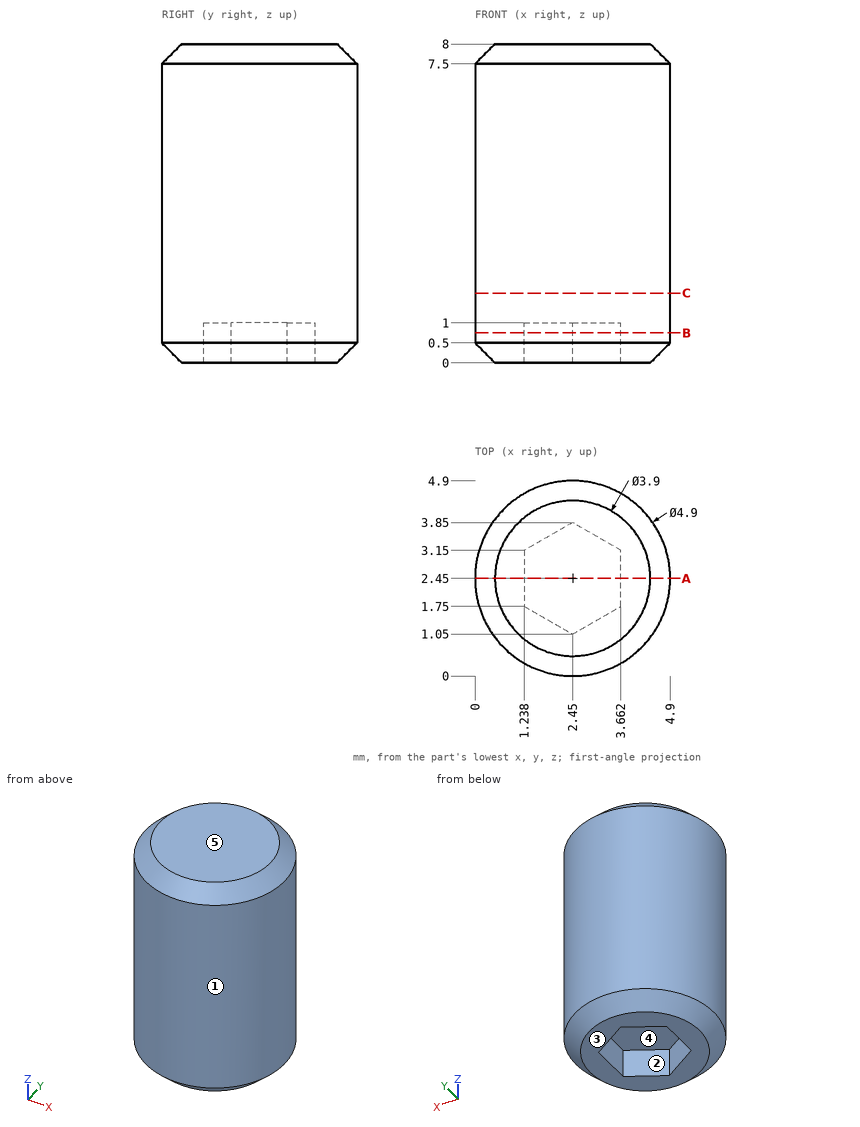
Job drawing, mm, ordinate dimensions from the low corner. One solid piece. A direction names the side the tool comes from. Coordinates: 2 decimals unless noted, no trailing zeros. Order: outer loops, then holes, each group sorted by start corner. A loop starts at its lowest first (then second) coordinate and runs counter-clockwise, first axis right, second up. Notation, with made-up numbers: (62.5, 39.25) -> (96.5, 39.25) arc R30 cw to (96.5, 77.25) -> close; hole circle Ø11 at (40.25, -7.5). An arc over 180 degrees is marked (long way). Return JSON: item names as keys, results as strings. Group by question number.
Item 1: Wall check: line 1 along X through (y, z) = (2.35, 1.75); line 2 along Z through (x, y) = (3.15, 1.85); line 3 along X through (y, z) = (1.25, 5.75) (1 decimal). Give the ranges that are in metal, low to high. Write a range as [from, to].
Item 2: Saw through at B-B on z = 0.75. Write the cut outline in (x, y).
Item 3: Saw through at C-C on z = 1.75. Write the cut outline in (x, y).
Item 4: Saw through at A-A on y = 2.45. Write the cut outline in (x, z).
Item 5: Tool access for the marked faces 4 and 5: list every direction of +Z, -Z, +X, -X, +Y, -Y with a clear straight run to the whole face (end or side of a thin tool).
Item 6: Pull direction Y, two halves, no side cores. Call the marked faces 1, 2 and 3: pulls with the +Y half, pulls with the -Y half, needs draft (parallel to the pull), parting line crosses it, or undercut.
Values found:
{
 "1": {"line 1": "x = [0, 4.9]", "line 2": "z = [1, 8]", "line 3": "x = [0.3, 4.6]"},
 "2": {"outline": "circle Ø4.9 at (2.45, 2.45); hole (1.24, 1.75) -> (2.45, 1.05) -> (3.66, 1.75) -> (3.66, 3.15) -> (2.45, 3.85) -> (1.24, 3.15) -> close"},
 "3": {"outline": "circle Ø4.9 at (2.45, 2.45)"},
 "4": {"outline": "(0, 0.5) -> (0.5, 0) -> (1.24, 0) -> (1.24, 1) -> (3.66, 1) -> (3.66, 0) -> (4.4, 0) -> (4.9, 0.5) -> (4.9, 7.5) -> (4.4, 8) -> (0.5, 8) -> (0, 7.5) -> close"},
 "5": {"face 4": "-Z", "face 5": "+Z, +X, -X, +Y, -Y"},
 "6": {"face 1": "parting line crosses it", "face 2": "undercut", "face 3": "needs draft"}
}
